```python
from build123d import *

# Parameters (mm, degrees)
SKETCH1_R           = 22.75
SKETCH1_R_2         = 12.75
BOSS_EXTRUDE1_DEPTH = 3
SKETCH2_R           = 12.75
BOSS_EXTRUDE2_DEPTH = 7
BOSS_EXTRUDE3_START = 3
BOSS_EXTRUDE3_DEPTH = 3
FILLET4_R           = 5
SKETCH4_R           = 2.25
CUT_EXTRUDE1_DEPTH  = 15
FILLET5_R           = 3
SKETCH6_R           = 2.25
BOSS_EXTRUDE4_DEPTH = 17
SKETCH7_R           = 26.5
CUT_EXTRUDE3_DEPTH  = 30


with BuildPart() as part:
    # Sketch1 → Boss-Extrude1 (new body)
    with BuildSketch(Plane(origin=(0, 0, 0), x_dir=(1, 0, 0), z_dir=(0, 1, 0))):
        with Locations(Location((0, 0, 0), (0, 0, 270))):
            Circle(SKETCH1_R)
        with Locations(Location((0, 0, 0), (0, 0, 270))):
            Circle(SKETCH1_R_2, mode=Mode.SUBTRACT)
    extrude(amount=BOSS_EXTRUDE1_DEPTH)

    # Sketch2 → Boss-Extrude2 (add)
    with BuildSketch(Plane(origin=(0, 3, 0), x_dir=(1, 0, 0), z_dir=(0, 1, 0))):
        with BuildLine():
            Line((17.75, 0), (17.75, 40))
            Line((17.75, 40), (-17.75, 40))
            Line((-17.75, 40), (-17.75, 0))
            ThreePointArc((-17.75, 0), (-14.209371907, -10.637492656), (-5, -17.03122133))
            ThreePointArc((-5, -17.03122133), (0, -17.75), (5, -17.03122133))
            ThreePointArc((5, -17.03122133), (14.209371907, -10.637492656), (17.75, 0))
        make_face()
        with Locations(Location((0, 0, 0), (0, 0, 270))):
            Circle(SKETCH2_R, mode=Mode.SUBTRACT)
    extrude(amount=BOSS_EXTRUDE2_DEPTH)

    # Sketch3 → Boss-Extrude3 (add)
    with BuildSketch(Plane.XZ.offset(-3).offset(BOSS_EXTRUDE3_START)):
        with BuildLine():
            Line((17.75, -40), (17.75, -14.230249471))
            ThreePointArc((17.75, -14.230249471), (0, -22.75), (-17.75, -14.230249471))
            Line((-17.75, -14.230249471), (-17.75, -40))
            Line((-17.75, -40), (17.75, -40))
        make_face()
    extrude(amount=-BOSS_EXTRUDE3_DEPTH)

    # Fillet4
    fillet4_edges = [part.edges().sort_by_distance(p)[0] for p in [
        (17.75, 5, -40),
        (-17.75, 5, -40),
    ]]
    fillet(fillet4_edges, radius=FILLET4_R)

    # Sketch4 → Cut-Extrude1 (cut)
    with BuildSketch(Plane(origin=(0, 10, 0), x_dir=(1, 0, 0), z_dir=(0, 1, 0))):
        with Locations(Location((10, 28.707521, 0), (0, 0, 270))):
            Circle(SKETCH4_R)
        with Locations(Location((-10, 28.707521, 0), (0, 0, 270))):
            Circle(SKETCH4_R)
    extrude(amount=-CUT_EXTRUDE1_DEPTH, mode=Mode.SUBTRACT)

    # Fillet5
    fillet5_edges = [part.edges().sort_by_distance(p)[0] for p in [
        (-17.75, 3, -7.115124735),
        (17.75, 3, -7.115124735),
        (0, 3, 17.75),
    ]]
    fillet(fillet5_edges, radius=FILLET5_R)

    # Sketch6 → Boss-Extrude4 (add)
    with BuildSketch(Plane(origin=(0, 0, 0), x_dir=(-1, 0, 0), z_dir=(0, -1, 0))):
        with BuildLine():
            Line((17.75, 22.7), (17.75, 35))
            ThreePointArc((17.75, 35), (16.285533906, 38.535533906), (12.75, 40))
            Line((12.75, 40), (-12.75, 40))
            ThreePointArc((-12.75, 40), (-16.285533906, 38.535533906), (-17.75, 35))
            Line((-17.75, 35), (-17.75, 22.7))
            Line((-17.75, 22.7), (17.75, 22.7))
        make_face()
        with Locations(Location((10, 28.707521, 0), (0, 0, 270))):
            Circle(SKETCH6_R, mode=Mode.SUBTRACT)
        with Locations(Location((-10, 28.707521, 0), (0, 0, 270))):
            Circle(SKETCH6_R, mode=Mode.SUBTRACT)
    extrude(amount=BOSS_EXTRUDE4_DEPTH)

    # Sketch7 → Cut-Extrude3 (cut)
    with BuildSketch(Plane(origin=(0, 0, 0), x_dir=(-1, 0, 0), z_dir=(0, -1, 0))):
        Circle(SKETCH7_R)
    extrude(amount=CUT_EXTRUDE3_DEPTH, mode=Mode.SUBTRACT)


solid = part.part
```
Part model, mm, in its own coordinate system. A direction names the side the tool comes from. Give positions to 0.01 mm unless a question says otherwise; leave off trailing zeros. Order: outer loops, then holes, each group sorted by start corner. A loop starts at its lowest first (then second) coordinate and runs counter-clockwise, first axis right, second up. Notation, with made-up numbers: (30.25, 15.5) - (65.25, 15.5) arc R13 cw to (65.25, 31.5) - close; hole circle Ø10 at (36, 17.5). An arc over 180 degrees is marked (long way). Use one line per item in the form item = value.
Item 1: Which spindle directions (+Z, -Z, +X, -X, +Y, -Y) get a long thin tool onto all of the face, cutting with end or side? Do faces 4 (the face through (0, 3, 21)), 5 (the face through (-0.2, -8.4, -26.5)), 6 (the face through (-16, -8, -22.7)). Say none if no direction does.
Solution:
face_4 = +Z, +Y
face_5 = +Z, -Y
face_6 = +Z, +X, -X, -Y
Item 2: Slice it at B-B on z = -1. Give the cut face in (x, y).
Solution:
outline = (-22.73, 0) - (-12.71, 0) - (-12.71, 10) - (-17.75, 10) - (-17.75, 6) arc R3 cw to (-20.75, 3) - (-22.73, 3) - close; (12.71, 0) - (22.73, 0) - (22.73, 3) - (20.75, 3) arc R3 cw to (17.75, 6) - (17.75, 10) - (12.71, 10) - close
Item 3: Probe probe 1 along Z at (x, y) = (10, 4.5); probe 2 along Y at (x, z) = (-10, -16); probe 3 along X at (y, z) = (-12.5, -24). List the from-to ranges inside material, lowest first. Write a range as from..to.
Solution:
probe_1 = -40..-30.96, -26.46..-7.91, 7.91..15.15
probe_2 = 0..10
probe_3 = -17.75..-11.24, 11.24..17.75
Item 4: Slice it at C-C on x = 0. Give the cut face in (y, z), and give its area (3 significant figures).
Solution:
outline = (-17, -40) - (10, -40) - (10, -12.75) - (0, -12.75) - (0, -26.5) - (-17, -26.5) - close; (0, 12.75) - (10, 12.75) - (10, 17.75) - (6, 17.75) arc R3 cw to (3, 20.75) - (3, 22.75) - (0, 22.75) - close
area = 569 mm2
Item 5: Pin check, flat tips, straight feed: pin 1 Ø3.5 at (x, z) = (10, -28.71) entering from +Y; pin 2 Ø4.5 at (x, y) = (16, -7.5) entering from +Z; pin 3 Ø1.5 at (y, z) = (0, -15.5) entering from -X; pin 4 Ø5 at (x, z) = (-12, -3) entering from -Y. Stop position of each tip, or through.
Solution:
pin_1 = through
pin_2 = -22.7
pin_3 = -17.75
pin_4 = 0
Item 6: Slice it at D-D on y = 5. Give the cut face in (x, z).
Solution:
outline = (-17.92, -14.01) arc R22.75 ccw to (-17.75, -14.23) - (-17.75, -35) arc R5 ccw to (-12.75, -40) - (12.75, -40) arc R5 ccw to (17.75, -35) - (17.75, -14.23) arc R22.75 ccw to (17.92, -14.01) - (17.92, 0) arc R17.92 ccw to (-17.92, 0) - close; hole circle Ø25.5 at (0, 0); hole circle Ø4.5 at (-10, -28.71); hole circle Ø4.5 at (10, -28.71)
Item 7: Two-plate mould, pull along Z, no slides. Class faces 1 (the face through (-0.72, 1.62, 22.74)), 2 (the face through (5, 0, -12)), 3 (the face through (9.901, -3.311, -30.955)): released by +Z, released by -Z, zero draft, split by the parting line, or undercut.
Solution:
face_1 = split by the parting line
face_2 = zero draft
face_3 = undercut
Item 8: Slice it at A-A on y = -14.75. Give the cut face in (x, z), and give its area (3 significant figures).
Solution:
outline = (-17.75, -35) arc R5 ccw to (-12.75, -40) - (12.75, -40) arc R5 ccw to (17.75, -35) - (17.75, -22.7) - (13.67, -22.7) arc R26.5 cw to (-13.67, -22.7) - (-17.75, -22.7) - close; hole circle Ø4.5 at (-10, -28.71); hole circle Ø4.5 at (10, -28.71)
area = 501 mm2
